Can you work these out from the model? Positions are in its coordinate system, mm. Give positions to 0.01 mm unless a question says otherwise; leave off trailing zeros. Write each loop counter-clockwise with the first axis right and the second up, starting at its lowest first coordinate (ties: lowest second). Pieces come first, ordered by that corner, then holes.
from build123d import *

# Parameters (mm, degrees)
SKETCH_W      = 60
SKETCH_H      = 25
EXTRUDE_DEPTH = 3
FILLET_R      = 3
SKETCH001_R   = 2
POCKET_DEPTH  = 3.001
FILLET001_R   = 1
FILLET002_R   = 0.4


with BuildPart() as part:
    # Sketch (on Sketch) → Extrude (new body)
    with BuildSketch(Plane.XY):
        with Locations((30, 12.5)):
            Rectangle(SKETCH_W, SKETCH_H)
    extrude(amount=EXTRUDE_DEPTH)

    # Fillet
    fillet_edges = [part.edges().sort_by_distance(p)[0] for p in [
        (0, 25, 1.5),
        (0, 0, 1.5),
        (60, 0, 1.5),
        (60, 25, 1.5),
    ]]
    fillet(fillet_edges, radius=FILLET_R)

    # Sketch001 (on Face5 of Fillet) → Pocket (cut, through all)
    with BuildSketch(Plane.XY.offset(3)):
        with Locations((6, 12.5)):
            Circle(SKETCH001_R)
    extrude(amount=-POCKET_DEPTH, mode=Mode.SUBTRACT)

    # Fillet001
    fillet001_edges = [part.edges().sort_by_distance(p)[0] for p in [
        (4, 12.5, 3),
        (4, 12.5, 0),
    ]]
    fillet(fillet001_edges, radius=FILLET001_R)

    # Fillet002
    fillet002_edges = [part.edges().sort_by_distance(p)[0] for p in [
        (60, 12.5, 3),
        (59.12132, 24.12132, 3),
        (30, 25, 3),
        (0.87868, 24.12132, 3),
        (0, 12.5, 3),
        (0.87868, 0.87868, 3),
        (30, 0, 3),
        (59.12132, 0.87868, 3),
        (59.12132, 0.87868, 0),
        (30, 0, 0),
        (0.87868, 0.87868, 0),
        (0, 12.5, 0),
        (0.87868, 24.12132, 0),
        (30, 25, 0),
        (59.12132, 24.12132, 0),
        (60, 12.5, 0),
    ]]
    fillet(fillet002_edges, radius=FILLET002_R)


solid = part.part
(1) Imagine slicing it at A-A, the plane x = 6. Write out the boundary of the cut face in (y, z).
Returned:
outline: (0, 0.4) arc R0.4 ccw to (0.4, 0) - (9.5, 0) arc R1 ccw to (10.5, 1) - (10.5, 2) arc R1 ccw to (9.5, 3) - (0.4, 3) arc R0.4 ccw to (0, 2.6) - close; (14.5, 1) arc R1 ccw to (15.5, 0) - (24.6, 0) arc R0.4 ccw to (25, 0.4) - (25, 2.6) arc R0.4 ccw to (24.6, 3) - (15.5, 3) arc R1 ccw to (14.5, 2) - close
(2) Imagine slicing it at B-B, the plane y = 12.5. Write out the boundary of the cut face in (x, z).
Returned:
outline: (0, 0.4) arc R0.4 ccw to (0.4, 0) - (3, 0) arc R1 ccw to (4, 1) - (4, 2) arc R1 ccw to (3, 3) - (0.4, 3) arc R0.4 ccw to (0, 2.6) - close; (8, 1) arc R1 ccw to (9, 0) - (59.6, 0) arc R0.4 ccw to (60, 0.4) - (60, 2.6) arc R0.4 ccw to (59.6, 3) - (9, 3) arc R1 ccw to (8, 2) - close
(3) If I drill on L1, parallel to Y at x = 6, z = 1.2; L2, parallel to Y at x = 47, z = 0.35; L3, parallel to X at y = 22.25, z = 0.75, over which ranges is the centre line in solid material (lowest first)?
Returned:
L1: y = 0 to 10.5, 14.5 to 25
L2: y = 0 to 25
L3: x = 0.01 to 59.99
(4) If we mould it in two halves opening along Y, with no side actions, what happens to faces 1 (the face through (5.74, 14.483, 1.507)), 2 (the face through (59.1, 0.86, 1.52)), 3 (the face through (30, 13, 0))? For each: +Y half, -Y half, draft (parallel to the pull), parting line (faces both ways), or undercut.
Returned:
face 1: undercut
face 2: -Y half
face 3: draft
